Verification items for this drawing (mm, ordinates from the low corner). A direction names the side the tool comes from. Round coordinates to 2 decimals unless told otherwise and drop trailing zeros. Loops run counter-clockwise (first coordinate to the right, second up) from the corner with the lowest first, then second, coordinate; pieces in that order, holes last. Notation, with made-up numbers: (33, -32.5) - (48, -32.5) arc R26 ccw to (48, -16.5) - close; hole circle Ø7 at (78, -14.5). An arc over 180 degrees is marked (long way). Answer in a Markdown table with one row per item. Add a question column.
(1) Cross-section at D-D on x = 29. Enter the section's corners in (y, z).
(2) Gauge pin test, flat ends, axial feed: pin 1 (3 mm diameter, centred on y = 18, z = 5.5, fed in from +X); pin 2 (2.5 mm diameter, centred on x = 5, z = 3, fed in from +Y); pin 3 (5 mm diameter, centred on y = 8, z = 5.5, fed in from -X). Record the tip position at first contact, or that the pin passes through.
(3) Access from +Z, -Z, +X, -X, +Y, -Y to the whole of each face (thin tool, end or side, straight path). Record for the marked faces 1, 2 and 3.
(4) Mould release check, pull along Y, two halves, no side actions. Record for the marked faces 4, 5, 6 and 7: +Y half, -Y half, draft (parallel to the pull), parting line (faces both ways), or undercut.
(5) Cross-section at B-B on z = 5. Enter the section's corners in (x, y), then the cut area to 3 significant figures.
(6) Cross-section at C-C on y = 21.5. Enter the section's corners in (x, z), then the cut area to 3 significant figures.
(7) Thickness scan on line 1 along Z through (x, y) = (5, 3.4); line 2 along Y through (x, z) = (40, 2.25); line 3 along X through (y, z) = (19.25, 9.25). Record the ranges inside material, lowest first.
(8) Cross-section at A-A on x = 40. Enter the section's corners in (y, z).
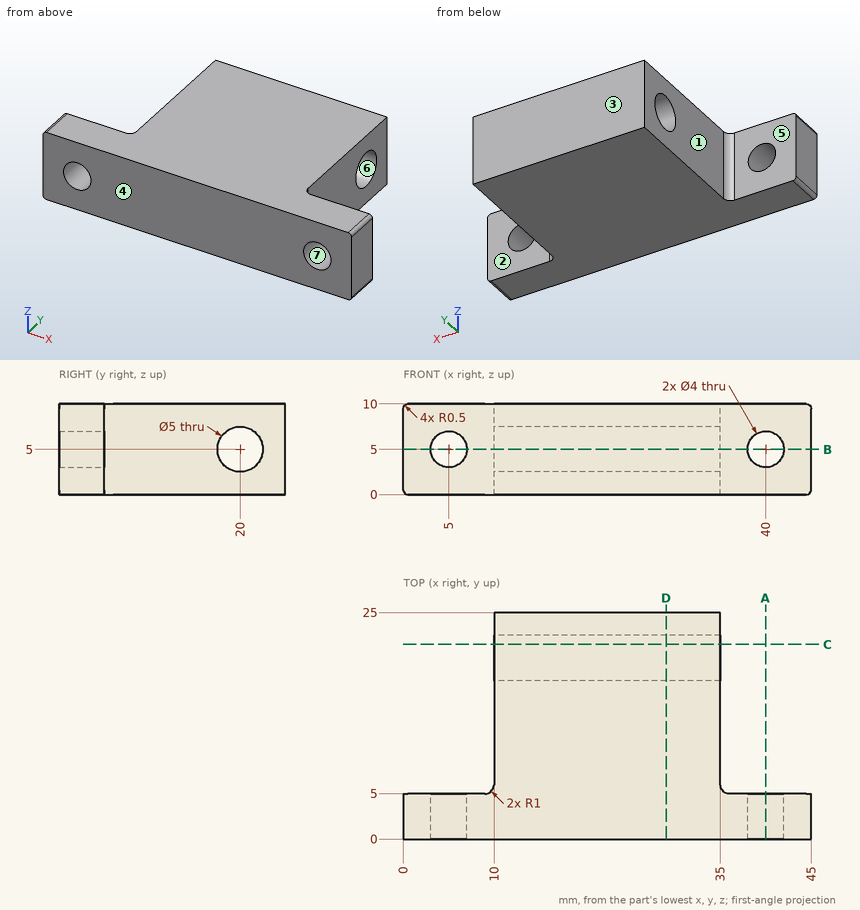
Answers:
| question | item | result |
|---|---|---|
| 1 | outline | (0, 0) - (25, 0) - (25, 10) - (0, 10) - close; hole circle Ø5 at (20, 5) |
| 2 | pin 1 | stops at x = 35 |
| 2 | pin 2 | stops at y = 5 |
| 2 | pin 3 | stops at x = 9.87 |
| 3 | face 1 | +Z, -Z, -X, +Y |
| 3 | face 2 | +Z, -Z, +X, +Y |
| 3 | face 3 | +Z, -Z, +X, -X, +Y |
| 4 | face 4 | -Y half |
| 4 | face 5 | +Y half |
| 4 | face 6 | undercut |
| 4 | face 7 | draft |
| 5 | outline | (0, 0) - (3, 0) - (3, 5) - (0, 5) - close; (7, 0) - (38, 0) - (38, 5) - (36, 5) arc R1 cw to (35, 6) - (35, 17.5) - (10, 17.5) - (10, 6) arc R1 cw to (9, 5) - (7, 5) - close; (10, 22.5) - (35, 22.5) - (35, 25) - (10, 25) - close; (42, 0) - (45, 0) - (45, 5) - (42, 5) - close |
| 5 | area | 560 mm^2 |
| 6 | outline | (10, 0) - (35, 0) - (35, 3) - (10, 3) - close; (10, 7) - (35, 7) - (35, 10) - (10, 10) - close |
| 6 | area | 150 mm^2 |
| 7 | line 1 | z = 0 to 3, 7 to 10 |
| 7 | line 2 | y = 0 to 5 |
| 7 | line 3 | x = 10 to 35 |
| 8 | outline | (0, 0) - (5, 0) - (5, 3) - (0, 3) - close; (0, 7) - (5, 7) - (5, 10) - (0, 10) - close |
